```python
from build123d import *

# Parameters (mm, degrees)
SKETCH_1_W      = 196.088
SKETCH_1_H      = 130.048
EXTRUDE_1_DEPTH = 157.48
SKETCH_3_W      = 25
SKETCH_3_H      = 35
EXTRUDE_2_DEPTH = 8
FILLET_2_R      = 12.5


with BuildPart() as part:
    # 草图1 → 凸台-拉伸1 (new body)
    with BuildSketch(Plane(origin=(0, 0, 0), x_dir=(1, 0, 0), z_dir=(0, 1, 0))):
        Rectangle(SKETCH_1_W, SKETCH_1_H)
    extrude(amount=EXTRUDE_1_DEPTH)

    # 草图3 → 凸台-拉伸2 (add)
    with BuildSketch(Plane(origin=(0, 157.48, 0), x_dir=(1, 0, 0), z_dir=(0, 1, 0))):
        with Locations((-85.544, -47.524)):
            Rectangle(SKETCH_3_W, SKETCH_3_H)
        with Locations((85.544, -47.524)):
            Rectangle(SKETCH_3_W, SKETCH_3_H)
    extrude(amount=EXTRUDE_2_DEPTH)

    # 圆角2
    fillet_2_edges = [part.edges().sort_by_distance(p)[0] for p in [
        (73.044, 161.48, 30.024),
        (98.044, 161.48, 30.024),
        (-98.044, 161.48, 30.024),
        (-73.044, 161.48, 30.024),
    ]]
    fillet(fillet_2_edges, radius=FILLET_2_R - 0.0001)  # a hair under: the kernel refuses the full size


solid = part.part
```
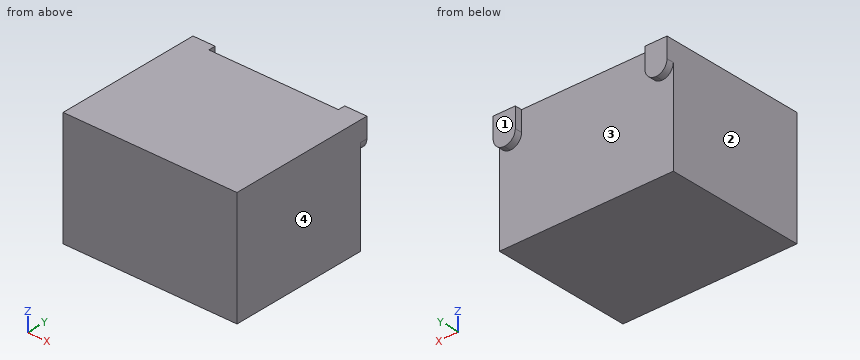
Geometry: final body of the model. Coordinates: model frame, mm. Face numbers are marked on the shaded views. Coordinates: 2 decimals unless noted, no trailing zeros. Loops run counter-clockwise (first coordinate to the right, second up) from the corner with the lowest first, then second, coordinate; pieces in that order, holes last. Notation, with made-up numbers: (16.25, 28.5) -> (63.25, 28.5) arc R23 ccw to (63.25, 44.5) -> close; hole circle Ø2 at (74, 31.5). An arc over 180 degrees is marked (long way). Use a Markdown table: item, result. Add a question column.
(1) Section query D-D, the plane x = -79.5. Return loops of the section in (y, z), plus the area to 3 significant figures.
(2) Mould query, pull axis X, two halves, no side actions, for the marked faces 1, 2, 3 and 4. Classes: pulls with the +X half, pulls with the -X half, needs draft (parallel to the pull), parting line crosses it, or undercut.
(3) Section query A-A, the plane z = 53. Return loops of the section in (x, y).
(4) Section query B-B, the plane x = 53. Return loops of the section in (y, z), plus the area to 3 significant figures.
(5) Pin query (flat end, axial travel): pin 1 Ø2 at (x, z) = (46, 37.5) entering from -Y; pin 2 Ø6 at (x, z) = (8.5, 29.5) entering from +Y. Return the tip coordinate at first contact, or that it passes through.
(6) Section query C-C, the plane z = -2.5. Return loops of the section in (x, y).
(7) Line query: line 1 along Y through (x, z) = (-33, -33.5). Output: solid intervals per line, ascending.
Answer:
| question | item | result |
|---|---|---|
| 1 | outline | (0, -65.02) -> (157.48, -65.02) -> (157.48, 31.58) -> (165.48, 31.58) -> (165.48, 65.02) -> (0, 65.02) -> close |
| 1 | area | 20,700 mm^2 |
| 2 | face 1 | needs draft |
| 2 | face 2 | pulls with the -X half |
| 2 | face 3 | undercut |
| 2 | face 4 | pulls with the +X half |
| 3 | outline | (-98.04, 0) -> (98.04, 0) -> (98.04, 165.48) -> (73.04, 165.48) -> (73.04, 157.48) -> (-73.04, 157.48) -> (-73.04, 165.48) -> (-98.04, 165.48) -> close |
| 4 | outline | (0, -65.02) -> (157.48, -65.02) -> (157.48, 65.02) -> (0, 65.02) -> close |
| 4 | area | 20,500 mm^2 |
| 5 | pin 1 | stops at y = 0 |
| 5 | pin 2 | stops at y = 157.48 |
| 6 | outline | (-98.04, 0) -> (98.04, 0) -> (98.04, 157.48) -> (-98.04, 157.48) -> close |
| 7 | line 1 | y = 0 to 157.48 |
